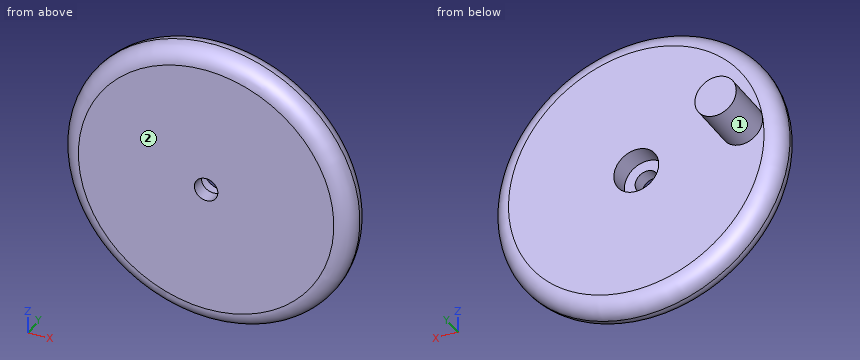
```python
from build123d import *

# Parameters (mm, degrees)
SKETCH1_R                      = 21
BOSS_EXTRUDE1_DEPTH            = 5
FILLET1_R                      = 2.5
SKETCH2_R                      = 3
BOSS_EXTRUDE2_DEPTH            = 7.5
CBORE_FOR_M3_SHCS1_D           = 3.4
CBORE_FOR_M3_SHCS1_CBORE_D     = 6.5
CBORE_FOR_M3_SHCS1_CBORE_DEPTH = 3


with BuildPart() as part:
    # Sketch1 → Boss-Extrude1 (new body)
    with BuildSketch(Plane(origin=(0, 0, 0), x_dir=(1, 0, 0), z_dir=(0, 1, 0))):
        with Locations(Location((0, 0, 0), (0, 0, 270))):
            Circle(SKETCH1_R)
    extrude(amount=BOSS_EXTRUDE1_DEPTH)

    # Fillet1
    fillet1_edges = [part.edges().sort_by_distance(p)[0] for p in [
        (0, 0, -21),
        (0, 5, -21),
    ]]
    fillet(fillet1_edges, radius=FILLET1_R - 0.0001)  # a hair under: the kernel refuses the full size

    # Sketch2 → Boss-Extrude2 (add)
    with BuildSketch(Plane(origin=(0, 5, 0), x_dir=(1, 0, 0), z_dir=(0, 1, 0))):
        with Locations(Location((-15.314964139, -2.387859588, 0), (0, 0, 188.862019992))):
            Circle(SKETCH2_R)
    extrude(amount=BOSS_EXTRUDE2_DEPTH)

    # CBORE for M3 SHCS1 (through all)
    with Locations(Plane(origin=(0, 5, 0), x_dir=(1, 0, 0), z_dir=(0, 1, 0))):
        with Locations((0, 0)):
            CounterBoreHole(CBORE_FOR_M3_SHCS1_D / 2, CBORE_FOR_M3_SHCS1_CBORE_D / 2, CBORE_FOR_M3_SHCS1_CBORE_DEPTH)


solid = part.part
```
Read the model definition and answer for the solid it produces. Units are mm, in the model's axes. Face numbers are marked on the shaded views. A direction names the side the tool comes from. Round coordinates to 2 decimals unless told otherwise and drop trailing zeros. Write each loop counter-clockwise with the first axis right and the second up, starting at its lowest first coordinate (ties: lowest second). Pieces come first, ordered by that corner, then holes. Notation, with made-up numbers: (30.25, 87.25) -> (73.25, 87.25) arc R23 ccw to (73.25, 125.25) -> close; hole circle Ø8 at (51.25, 71.25). An arc over 180 degrees is marked (long way). Answer in a Markdown table with one row per item. Add a question column.
1) Given P1, Ø3, axis at y = 5.5, z = 2, coming from the +X side; P2, Ø6, axis at x = -12, y = 9, coming from the -Z side; P3, Ø5, axis at x = 0, z = 1.5, coming from the +Y side, each flat-ended and moving along its own axis, determine where each tip first touches the part or whether it passes through.
2) Find section D-D, the plane y = 11.5. Determine the outline of the cut face in (x, z).
3) Consider line 1 (Y direction, x = -12, z = -3.5); line 2 (X direction, y = 9, z = 2.5); line 3 (Z direction, x = 1.5, y = 2.75). Determine where each line is inside the solid, lowest interval first.
4) Find section C-C, the plane y = 3. Determine the outline of the cut face in (x, z).
5) Which of the six approach directions +Z, -Z, +X, -X, +Y, -Y give full straight-line access (tool end or side, diameter ignored) to the marked faces 1 and 2?
Findings below:
| question | item | result |
|---|---|---|
| 1 | P1 | x = 20.41 |
| 1 | P2 | z = -0.6 |
| 1 | P3 | y = 5 |
| 2 | outline | circle Ø6 at (-15.31, 2.39) |
| 3 | line 1 | 0 to 5 |
| 3 | line 2 | -18.31 to -12.32 |
| 3 | line 3 | -20.93 to -2.88, 2.88 to 20.93 |
| 4 | outline | circle Ø41.9 at (0, 0); hole circle Ø6.5 at (0, 0) |
| 5 | face 1 | +Y |
| 5 | face 2 | +Z, -Z, +X, -X, -Y |
